from build123d import *

# Parameters (mm, degrees)
F1_DEPTH = 500
F2_W     = 14
F2_H     = 150
F3_DEPTH = 200.001
F4_W     = 150
F4_H     = 14
F5_DEPTH = 200.001


with BuildPart() as f1:
    # F0 (on Front) → F1 (new body)
    with BuildSketch(Plane.XZ):
        with BuildLine():
            ThreePointArc((100, 80), (94.142136, 94.142136), (80, 100))
            Line((80, 100), (-80, 100))
            ThreePointArc((-80, 100), (-94.142136, 94.142136), (-100, 80))
            Line((-100, 80), (-100, -80))
            ThreePointArc((-100, -80), (-94.142136, -94.142136), (-80, -100))
            Line((-80, -100), (80, -100))
            ThreePointArc((80, -100), (94.142136, -94.142136), (100, -80))
            Line((100, -80), (100, 80))
        make_face()
        with BuildLine():
            Line((-80, 90), (80, 90))
            ThreePointArc((80, 90), (87.071068, 87.071068), (90, 80))
            Line((90, 80), (90, -80))
            ThreePointArc((90, -80), (87.071068, -87.071068), (80, -90))
            Line((80, -90), (-80, -90))
            ThreePointArc((-80, -90), (-87.071068, -87.071068), (-90, -80))
            Line((-90, -80), (-90, 80))
            ThreePointArc((-90, 80), (-87.071068, 87.071068), (-80, 90))
        make_face(mode=Mode.SUBTRACT)
    extrude(amount=F1_DEPTH)

    # F2 (on face) → F3 (cut, through all)
    with BuildSketch(Plane.XY.offset(100)):
        with Locations((0, -75)):
            Rectangle(F2_W, F2_H)
    extrude(amount=-F3_DEPTH, mode=Mode.SUBTRACT)

    # F4 (on face) → F5 (cut, through all)
    with BuildSketch(Plane.YZ.offset(100)):
        with Locations((-75, 0)):
            Rectangle(F4_W, F4_H)
    extrude(amount=-F5_DEPTH, mode=Mode.SUBTRACT)


solid = f1.part
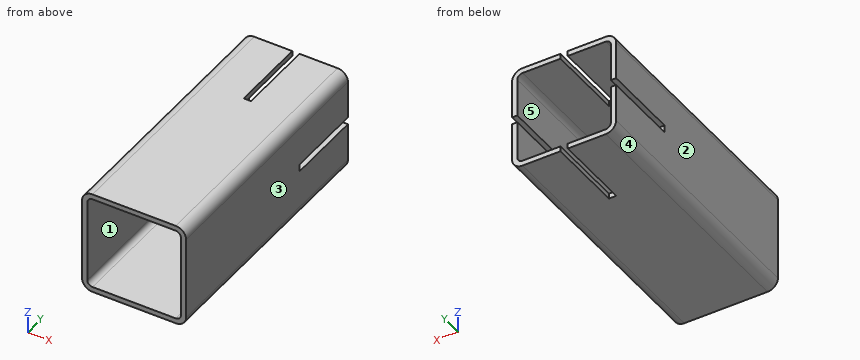
Verification items for the finished model (mm, model axes). Face numbers are marked on the shaded views. A direction names the side the tool comes from. Give positions to 0.01 mm unless a question says otherwise; leave off trailing zeros. Loops run counter-clockwise (first coordinate to the right, second up) from the corner with the lowest first, then second, coordinate; pieces in that order, holes last.
1) Draft check along X on the marked faces 1, 2 and 3. Enter one of: pulls with the +X half, pulls with the -X half, needs draft (parallel to the pull), parting line crosses it, or undercut.
2) Depth check by flat-ended pin: pin 1 Ø3 at (y, z) = (-39, 96) entering from -X (3 decimals); pin 2 Ø3 at (y, z) = (-102, -93.5) entering from +X; pin 3 Ø3 at (x, z) = (-95, -0.5) entering from +Y. Enter the tip coordinate at first touch or a pass-through.
3) Set-up check for the marked faces 4 and 5: record each of +Z, -Z, +X, -X, +Y, -Y from which the full face is reachable in a straight line by a thin tool's end or side.
4) Sectioned sample at B-B, the plane y = -80. Count the separate pieces of the cut face and the enclosed holes in it, then the cut area to 3 significant figures.
5) Sectioned sample at D-D, the plane y = -367. Enter the section's corners in (x, z).
6) Sectioned sample at A-A, the plane x = 18.5. Enter the section's corners in (y, z), then the cut area to 3 significant figures.
7) Thickness scan on line 1 along X through (y, z) = (-415.5, 22.5); line 2 along Z through (x, y) = (84.5, -172). Record the ranges inside material, lowest first.
8) Sectioned sample at C-C, the plane z = 52.5. Enter the section's corners in (x, y).
Answers:
1. face 1: undercut
1. face 2: pulls with the -X half
1. face 3: pulls with the +X half
2. pin 1: stops at x = -93.775
2. pin 2: stops at x = 96
2. pin 3: stops at y = -150
3. face 4: -Z, -X, +Y, -Y
3. face 5: +Y, -Y
4. separate pieces: 4
4. enclosed holes: 0
4. area: 6,780 mm2
5. outline: (-100, -80) arc R20 ccw to (-80, -100) - (80, -100) arc R20 ccw to (100, -80) - (100, 80) arc R20 ccw to (80, 100) - (-80, 100) arc R20 ccw to (-100, 80) - close; hole (-90, -80) arc R10 ccw to (-80, -90) - (80, -90) arc R10 ccw to (90, -80) - (90, 80) arc R10 ccw to (80, 90) - (-80, 90) arc R10 ccw to (-90, 80) - close
6. outline: (-500, -100) - (0, -100) - (0, -90) - (-500, -90) - close; (-500, 90) - (0, 90) - (0, 100) - (-500, 100) - close
6. area: 10,000 mm2
7. line 1: x = -100 to -90, 90 to 100
7. line 2: z = -99.49 to -88.93, 88.93 to 99.49
8. outline: (-100, -500) - (-90, -500) - (-90, 0) - (-100, 0) - close; (90, -500) - (100, -500) - (100, 0) - (90, 0) - close
